```python
from build123d import *

# Parameters (mm, degrees)
F0_W     = 35
F0_H     = 25
F1_DEPTH = 3
F2_R     = 2


with BuildPart() as f1:
    # F0 (on Top) → F1 (new body)
    with BuildSketch(Plane.XY):
        with Locations((-1.5, 0)):
            Rectangle(F0_W, F0_H)
        with BuildLine():
            ThreePointArc((-5.291503, 1.5), (0.757211, 5.447626), (5.5, 0))
            ThreePointArc((5.5, 0), (0.757211, -5.447626), (-5.291503, -1.5))
            Line((-5.291503, -1.5), (-9.291503, -1.5))
            Line((-9.291503, -1.5), (-9.291503, 1.5))
            Line((-9.291503, 1.5), (-5.291503, 1.5))
        make_face(mode=Mode.SUBTRACT)
    extrude(amount=F1_DEPTH)

    # F2
    f2_edges = [f1.edges().sort_by_distance(p)[0] for p in [
        (-19, -12.5, 1.5),
        (16, -12.5, 1.5),
        (16, 12.5, 1.5),
        (-19, 12.5, 1.5),
    ]]
    fillet(f2_edges, radius=F2_R)


solid = f1.part
```
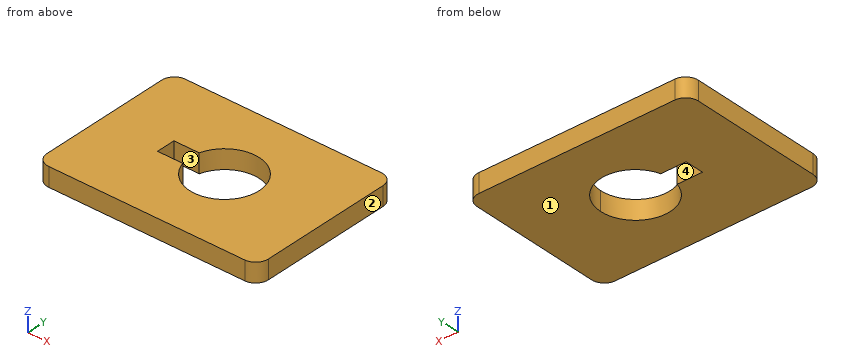
Work out the finished part from the listing and answer in its coordinate system (mm). Face numbers are marked on the shaded views. Give positions to 0.01 mm unless a question says otherwise; leave off trailing zeros. Order: outer loops, then holes, each group sorted by start corner. A loop starts at its lowest first (then second) coordinate and runs counter-clockwise, first axis right, second up. Notation, with made-up numbers: (-9.5, -3) -> (7.5, -3) arc R26 cw to (7.5, 26) -> close; hole circle Ø2 at (63, -15.75). An arc over 180 degrees is marked (long way). Answer as CSV lines item,"result". Start each with the question number.
(1) Section C-C, the plane z = 1.65 is taken. Write down the section's boundary in (x, y).
(2) Section B-B, the plane y = 4 is taken. Write down the section's boundary in (x, z), plus the area to 3 significant figures.
(3) Section A-A, the plane x = -8.5 is taken. Write down the section's boundary in (y, z).
(4) This flat-tipped pin is pushed along its axis until it touches: pin 1 Ø4 at (x, y) = (-13, -2) entering from -Z. Where does it stop, or does it pass through?
(5) For a pull along X with two mould halves and no side action, classify the marked faces 1, 2, 3 and 4 as released by +X, released by -X, zero draft, split by the parting line, or undercut.
(6) Consider line 1 along Y through (x, z) = (0, 2.6); line 2 along Y through (x, z) = (-7, 1.1); line 3 along X through (y, z) = (0.75, 2.2). Determine where each line is inside the solid, lowest interval first.
Entries:
1,outline,"(-19, -10.5) arc R2 ccw to (-17, -12.5) -> (14, -12.5) arc R2 ccw to (16, -10.5) -> (16, 10.5) arc R2 ccw to (14, 12.5) -> (-17, 12.5) arc R2 ccw to (-19, 10.5) -> close; hole (-9.29, -1.5) -> (-5.29, -1.5) arc R5.5 ccw (long way) to (-5.29, 1.5) -> (-9.29, 1.5) -> close"
2,outline,"(-19, 0) -> (-3.77, 0) -> (-3.77, 3) -> (-19, 3) -> close; (3.77, 0) -> (16, 0) -> (16, 3) -> (3.77, 3) -> close"
2,area,"82.4 mm²"
3,outline,"(-12.5, 0) -> (-1.5, 0) -> (-1.5, 3) -> (-12.5, 3) -> close; (1.5, 0) -> (12.5, 0) -> (12.5, 3) -> (1.5, 3) -> close"
4,pin 1,"z = 0"
5,face 1,"zero draft"
5,face 2,"released by +X"
5,face 3,"undercut"
5,face 4,"undercut"
6,line 1,"-12.5 to -5.5, 5.5 to 12.5"
6,line 2,"-12.5 to -1.5, 1.5 to 12.5"
6,line 3,"-19 to -9.29, 5.45 to 16"
